from build123d import *

# Parameters (mm, degrees)
F2_R      = 1.5
F3_DEPTH  = 16
F2_R_2    = 2.75
F3_FACE_R = 1.5
F4_DEPTH  = 3
F5_SIZE   = 0.3
F7_DEPTH  = 1.3


with BuildPart() as f3:
    # F2 (on Top) → F3 (new body)
    with BuildSketch(Plane.XY):
        Circle(F2_R)
    extrude(amount=-F3_DEPTH)

    # F2 (on Top) + F3_face (on face) → F4 (join)
    with BuildSketch(Plane.XY):
        Circle(F2_R_2)
        Circle(F2_R, mode=Mode.SUBTRACT)
    with BuildSketch(Plane.XY):
        Circle(F3_FACE_R)
    extrude(amount=F4_DEPTH)

    # F5
    f5_edges = [f3.edges().sort_by_distance(p)[0] for p in [
        (-1.5, 0, -16),
        (-2.75, 0, 3),
    ]]
    chamfer(f5_edges, length=F5_SIZE)

    # F6 (on face) → F7 (cut)
    with BuildSketch(Plane.XY.offset(3)):
        Polygon((1.25, -0.7216878365), (1.25, 0.7216878365), (0, 1.443375673), (-1.25, 0.7216878365), (-1.25, -0.7216878365), (0, -1.443375673), align=None)
    extrude(amount=-F7_DEPTH, mode=Mode.SUBTRACT)


solid = f3.part
The listing builds one solid part. Answer for the finished solid, in the listing's coordinates (mm). A direction names the side the tool comes from. Coordinates: 2 decimals unless noted, no trailing zeros. Order: outer loops, then holes, each group sorted by start corner. A loop starts at its lowest first (then second) coordinate and runs counter-clockwise, first axis right, second up.
Q1. A cutting plane is placed at A-A, the plane y = 0. Write down the section's boundary in (x, z).
Q2. A cutting plane is placed at B-B, the plane z = -13.25. Write down the section's boundary in (x, y).
Q3. Consider line 1 (Z direction, x = -1.8, y = 1.05); line 2 (X direction, y = 0.4, z = -7.75); line 3 (X direction, y = -0.1, z = -10.25). Determine where each line is inside the solid, lowest interval first.
Q4. Given P1, Ø3, axis at x = -0.5, y = 2, coming from the -Z side; P2, Ø0.6, axis at y = 0.5, z = 2.5, coming from the -X side; P3, Ø1.2, axis at x = 0, y = 0, coming from the +Z side, each flat-ended and moving along its own axis, determine where each tip first touches the part or whether it passes through.
Q5. Which of the six approach directions +Z, -Z, +X, -X, +Y, -Y give full straight-line access (tool end or side, diameter ignored) to faces 4 (the face through (1.1, -1.1, 3)), 5 (the face through (-1.25, 0, 2)), 6 (the face through (1.2, -1.2, 0))?
Q6. For a pull along Y with two mould halves and no side action, classify faces 1 (the face through (1.25, 0, 2)), 2 (the face through (0, 0, -16)), 3 (the face through (-0.596, -2.685, 1.331)) as pulls with the +Y half, pulls with the -Y half, needs draft (parallel to the pull), parting line crosses it, or undercut.
Answers follow:
1. outline: (-2.75, 0) - (-1.5, 0) - (-1.5, -15.7) - (-1.2, -16) - (1.2, -16) - (1.5, -15.7) - (1.5, 0) - (2.75, 0) - (2.75, 2.7) - (2.45, 3) - (1.25, 3) - (1.25, 1.7) - (-1.25, 1.7) - (-1.25, 3) - (-2.45, 3) - (-2.75, 2.7) - close
2. outline: circle Ø3 at (0, 0)
3. line 1: z = 0 to 3
3. line 2: x = -1.45 to 1.45
3. line 3: x = -1.5 to 1.5
4. P1: stops at z = -16
4. P2: stops at x = -2.74
4. P3: stops at z = 1.7
5. face 4: +Z, +X, -X, +Y, -Y
5. face 5: +Z
5. face 6: -Z
6. face 1: undercut
6. face 2: needs draft
6. face 3: parting line crosses it
